```python
from build123d import *

# Parameters (mm, degrees)
SKETCH1_W           = 165
SKETCH1_H           = 45
SKETCH1_R           = 1.5
SKETCH1_W_2         = 6.35
SKETCH1_H_2         = 10
BOSS_EXTRUDE1_DEPTH = 6.35


with BuildPart() as part:
    # Sketch1 → Boss-Extrude1 (new body)
    with BuildSketch(Plane(origin=(0, 0, 0), x_dir=(1, 0, 0), z_dir=(0, 1, 0))):
        with Locations((82.5, 22.5)):
            Rectangle(SKETCH1_W, SKETCH1_H)
        with Locations(Location((14.721825407, 30.278174593, 0), (0, 0, 270))):
            Circle(SKETCH1_R, mode=Mode.SUBTRACT)
        with Locations(Location((14.721825407, 14.721825407, 0), (0, 0, 270))):
            Circle(SKETCH1_R, mode=Mode.SUBTRACT)
        with Locations(Location((30.278174593, 30.278174593, 0), (0, 0, 270))):
            Circle(SKETCH1_R, mode=Mode.SUBTRACT)
        with Locations(Location((30.278174593, 14.721825407, 0), (0, 0, 270))):
            Circle(SKETCH1_R, mode=Mode.SUBTRACT)
        with Locations(Location((41.5, 22.5, 0), (0, 0, 270))):
            Circle(SKETCH1_R, mode=Mode.SUBTRACT)
        with Locations(Location((69.5, 22.5, 0), (0, 0, 270))):
            Circle(SKETCH1_R, mode=Mode.SUBTRACT)
        with Locations(Location((155, 7.5, 0), (0, 0, 270))):
            Circle(SKETCH1_R, mode=Mode.SUBTRACT)
        with Locations(Location((155, 37.5, 0), (0, 0, 270))):
            Circle(SKETCH1_R, mode=Mode.SUBTRACT)
        with Locations(Location((35, 37.5, 0), (0, 0, 270))):
            Circle(SKETCH1_R, mode=Mode.SUBTRACT)
        with Locations(Location((35, 7.5, 0), (0, 0, 270))):
            Circle(SKETCH1_R, mode=Mode.SUBTRACT)
        with Locations((84.675, 22.5)):
            Rectangle(SKETCH1_W_2, SKETCH1_H_2, mode=Mode.SUBTRACT)
        with Locations((154.325, 22.5)):
            Rectangle(SKETCH1_W_2, SKETCH1_H_2, mode=Mode.SUBTRACT)
    extrude(amount=BOSS_EXTRUDE1_DEPTH)


solid = part.part
```
Input: part model. Units: mm. Frame: model coordinates. A direction names the side the tool comes from. Round coordinates to 2 decimals unless told otherwise and drop trailing zeros. Order: outer loops, then holes, each group sorted by start corner. A loop starts at its lowest first (then second) coordinate and runs counter-clockwise, first axis right, second up. Notation, with made-up numbers: (-32.75, -30.75) - (-3.75, -30.75) arc R19 cw to (-3.75, -14.75) - close; hole circle Ø5 at (21.25, 14). An arc over 180 degrees is marked (long way). One line per question, with ' | ' between items. Start each with the question number.
1) Cut plane A-A, the plane z = -37.5. Return the cut outline in (x, y).
2) Cut plane D-D, the plane x = 155. Return the cut outline in (y, z), then the cut area to 3 significant figures.
3) Pull-direction query (Z, two-part tool) for faces 1 (the flat face through (165, 3, -22)), 2 (the flat face through (81, 3, 0)), 3 (the cylindrical face through (70.987, 3.131, -22.695)), 4 (the cylindrical face through (33.536, 3.131, -7.825)); classes: +Z half, -Z half, draft (parallel to the pull), parting line (faces both ways), or undercut.
4) Cut plane B-B, the plane x = 35. Return the cut outline in (y, z), then the cut area to 3 significant figures.
5) Set-up query: faces 5 (the flat face through (154, 3, -17.5)), 6 (the flat face through (81, 0, -23)). Return all of +Z, -Z, +X, -X, +Y, -Y with unobstructed straight access to the full face (end or side cutting, diameter ignored); none if empty.
6) Cut plane C-C, the plane z = -22.5. Return the cut outline in (x, y).
7) Ray query, probe 1 along X at (y, z) = (4.5, -22.5); probe 2 along X at (y, z) = (4.25, -37.5); probe 3 along X at (y, z) = (3.5, -25). Return the intervals inside material, ascending.
Worked out:
1) outline: (0, 0) - (33.5, 0) - (33.5, 6.35) - (0, 6.35) - close; (36.5, 0) - (153.5, 0) - (153.5, 6.35) - (36.5, 6.35) - close; (156.5, 0) - (165, 0) - (165, 6.35) - (156.5, 6.35) - close
2) outline: (0, -45) - (6.35, -45) - (6.35, -39) - (0, -39) - close; (0, -36) - (6.35, -36) - (6.35, -27.5) - (0, -27.5) - close; (0, -17.5) - (6.35, -17.5) - (6.35, -9) - (0, -9) - close; (0, -6) - (6.35, -6) - (6.35, 0) - (0, 0) - close | area: 184 mm^2
3) face 1: draft | face 2: +Z half | face 3: undercut | face 4: undercut
4) outline: (0, -45) - (6.35, -45) - (6.35, -39) - (0, -39) - close; (0, -36) - (6.35, -36) - (6.35, -9) - (0, -9) - close; (0, -6) - (6.35, -6) - (6.35, 0) - (0, 0) - close | area: 248 mm^2
5) face 5: +Y, -Y | face 6: +Z, -Z, +X, -X, -Y
6) outline: (0, 0) - (40, 0) - (40, 6.35) - (0, 6.35) - close; (43, 0) - (68, 0) - (68, 6.35) - (43, 6.35) - close; (71, 0) - (81.5, 0) - (81.5, 6.35) - (71, 6.35) - close; (87.85, 0) - (151.15, 0) - (151.15, 6.35) - (87.85, 6.35) - close; (157.5, 0) - (165, 0) - (165, 6.35) - (157.5, 6.35) - close
7) probe 1: x = 0 to 40, 43 to 68, 71 to 81.5, 87.85 to 151.15, 157.5 to 165 | probe 2: x = 0 to 33.5, 36.5 to 153.5, 156.5 to 165 | probe 3: x = 0 to 81.5, 87.85 to 151.15, 157.5 to 165
